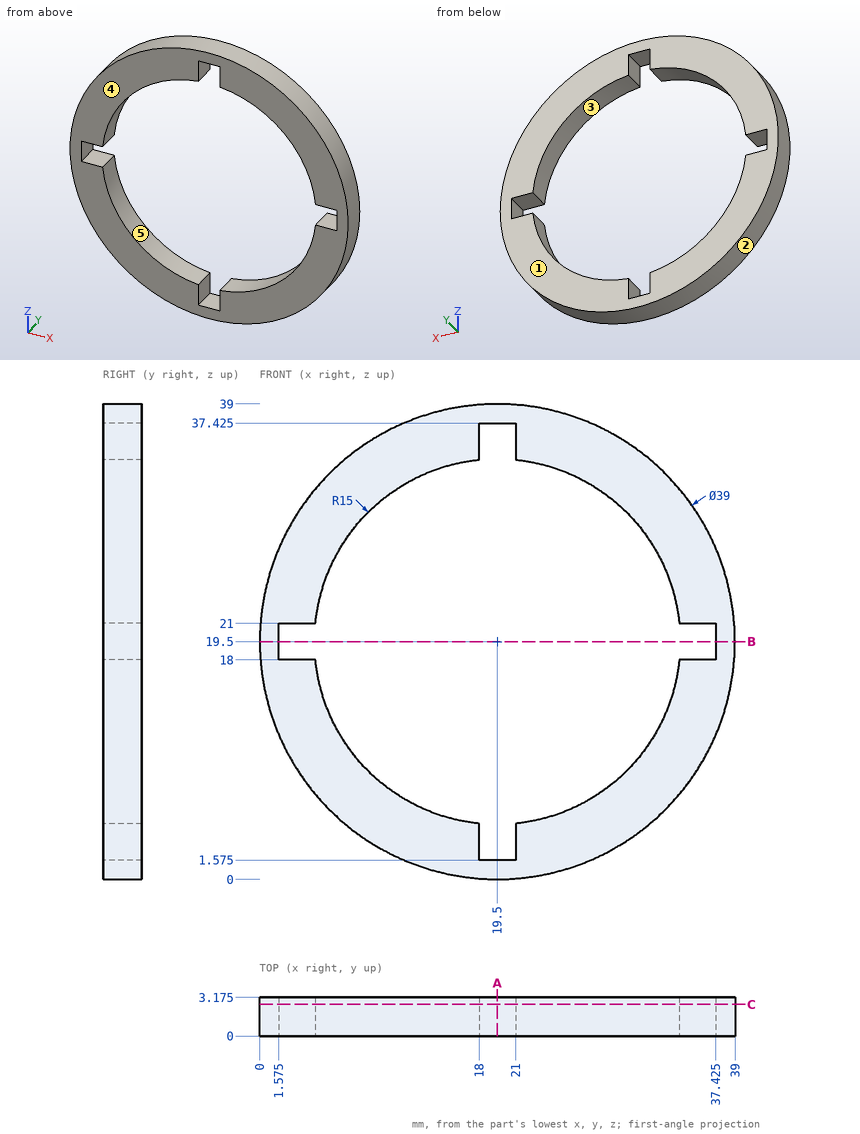
The drawing under review shows one solid part. Ordinate dimensions are in mm from its lowest x, y, z. A direction names the side the tool comes from. Round coordinates to 2 decimals unless told otherwise and drop trailing zeros. Order: outer loops, then holes, each group sorted by start corner. A loop starts at its lowest first (then second) coordinate and runs counter-clockwise, first axis right, second up. Notation, with made-up numbers: (-38, 81.5) -> (10, 81.5) arc R31 cw to (10, 115.5) -> close; hole circle Ø5 at (19, 37). An arc over 180 degrees is marked (long way). Use a Markdown table: item, result.
Q1. We need section B-B on z = 19.5. Write out the cut boundary in (x, y) (1 decimal), then the cut area to 3 significant figures.
Values:
| item | result |
|---|---|
| outline | (0, 0) -> (1.6, 0) -> (1.6, 3.2) -> (0, 3.2) -> close; (37.4, 0) -> (39, 0) -> (39, 3.2) -> (37.4, 3.2) -> close |
| area | 10.0 mm^2 |
Q2. Clearance check with flat-ended pins moving along their axes: P1, Ø1.5, axis at x = 20, y = 2, coming from the -Z side; P2, Ø6, axis at x = 15, z = 28.5, coming from the +Y side; P3, Ø1.5, axis at x = 3, y = 1, coming from the -Z side; P4, Ø0.9, axis at x = 2.5, y = 1.5, coming from the +Z side. State where each tip first meets the part, or that it passes through.
Values:
| item | result |
|---|---|
| P1 | stops at z = 0 |
| P2 | passes through |
| P3 | stops at z = 8 |
| P4 | stops at z = 29.81 |
Q3. We need section A-A on x = 19.5. Write out the cut boundary in (y, z) (1 decimal), then the cut area to 3 significant figures.
Values:
| item | result |
|---|---|
| outline | (0, 0) -> (3.2, 0) -> (3.2, 1.6) -> (0, 1.6) -> close; (0, 37.4) -> (3.2, 37.4) -> (3.2, 39) -> (0, 39) -> close |
| area | 10.0 mm^2 |
Q4. Mouldability with a two-part tool opening along Z and no side actions: class the marked faces 1, 2 and 3 as +Z half, -Z half, draft (parallel to the pull), parting line (faces both ways), or undercut.
Values:
| item | result |
|---|---|
| face 1 | draft |
| face 2 | parting line |
| face 3 | undercut |
Q5. For line 1 (Z direction, x = 9.5, y = 2.3); line 2 (X direction, y = 0.6, z = 14.5); line 3 (X direction, y = 0.95, z = 10.5), list the stretches that pass through material, from the lowest coordinate up.
Values:
| item | result |
|---|---|
| line 1 | z = 2.76 to 8.32, 30.68 to 36.24 |
| line 2 | x = 0.65 to 5.36, 33.64 to 38.35 |
| line 3 | x = 2.2 to 7.5, 31.5 to 36.8 |
Q6. Tool access review of the marked faces 4 and 5: name each direction out of +Z, -Z, +X, -X, +Y, -Y from which nothing blocks a thin tool from reaching the whole face with its end or side.
Values:
| item | result |
|---|---|
| face 4 | +Z, -Z, +X, -X, -Y |
| face 5 | +Y, -Y |
Q7. We need section C-C on y = 2.6. Write out the cut boundary in (x, z) (1 decimal).
Values:
| item | result |
|---|---|
| outline | circle Ø39 at (19.5, 19.5); hole (1.6, 18) -> (4.6, 18) arc R15 ccw to (18, 4.6) -> (18, 1.6) -> (21, 1.6) -> (21, 4.6) arc R15 ccw to (34.4, 18) -> (37.4, 18) -> (37.4, 21) -> (34.4, 21) arc R15 ccw to (21, 34.4) -> (21, 37.4) -> (18, 37.4) -> (18, 34.4) arc R15 ccw to (4.6, 21) -> (1.6, 21) -> close |
